For this review, take the finished solid that the model builds, in its own axes (mm). Give positions to 0.01 mm unless a question says otherwise; leave off trailing zeros. Loops run counter-clockwise (first coordinate to the right, second up) from the corner with the lowest first, then second, coordinate; pieces in that order, holes last. Notation, with made-up numbers: (-13.5, -7.75) -> (18.5, -7.75) arc R10 ccw to (18.5, 4.25) -> close; hole circle Ø8 at (37, 22.25). An arc over 180 degrees is marked (long way). Answer as CSV lines item,"result". Start each with the question number.
Item 1: For L1, parallel to Z at x = 136.5, y = 20.25; L2, parallel to Z at x = 135, y = 7.5; L3, parallel to Z at x = 72, y = 15, list the stretches that pass through material, from the lowest coordinate up. Write a range as from..to.
Item 2: Clearance check with flat-ended pins moving along their axes: P1, Ø0.8, axis at x = 211, y = 1, coming from the -Z side; P2, Ø4, axis at x = 289, z = 70, coming from the +Y side; P3, Ø0.5, axis at x = 345.5, y = 28.5, coming from the +Z side. State where each tip first meets the part, or that it passes through.
Item 3: The part is to be moulded in two halves that separate along Z. For faces 1 (the face through (303, 2.02, 60)), 2 (the face through (0, 15, 59)), 3 (the face through (303, 27.98, 60)), say which applies: +Z half, -Z half, draft (parallel to the pull), parting line (faces both ways), or undercut.
Item 4: Add section A-A on z = 28.5. State the section outline as (x, y) points, plus the area to 3 significant figures.
```python
from build123d import *

# Parameters (mm, degrees)
SKETCH1_W           = 598.4875
SKETCH1_H           = 30
BOSS_EXTRUDE1_DEPTH = 119.5
FILLET1_R           = 2
CUT_EXTRUDE1_REACH  = 613.038
FILLET2_R           = 0.5
CUT_EXTRUDE2_REACH  = 613.038
SKETCH3_W           = 98.3
SKETCH3_H           = 2.02
FILLET3_R           = 0.5


with BuildPart() as part:
    # Sketch1 → Boss-Extrude1 (new body)
    with BuildSketch(Plane.XY):
        with Locations((299.24375, 15)):
            Rectangle(SKETCH1_W, SKETCH1_H)
    extrude(amount=BOSS_EXTRUDE1_DEPTH)

    # Fillet1
    fillet1_edges = [part.edges().sort_by_distance(p)[0] for p in [
        (299.24375, 0, 119.5),
        (299.24375, 0, 0),
        (299.24375, 30, 0),
        (299.24375, 30, 119.5),
    ]]
    fillet(fillet1_edges, radius=FILLET1_R)

    # Sketch2 → Cut-Extrude1 (cut, up to next)
    with BuildSketch(Plane(origin=(598.4875, 0, 0), x_dir=(0, 0, -1), z_dir=(1, 0, 0)), mode=Mode.PRIVATE) as cut_extrude1_sk1:
        with BuildLine():
            Line((-119.5, 19.4), (-119.5, 10.6))
            Line((-119.5, 10.6), (-117.978098197, 10.6))
            ThreePointArc((-117.978098197, 10.6), (-117.624544806, 10.453553391), (-117.478098197, 10.1))
            Line((-117.478098197, 10.1), (-117.478098197, 6.87))
            ThreePointArc((-117.478098197, 6.87), (-117.331651588, 6.516446609), (-116.978098197, 6.37))
            Line((-116.978098197, 6.37), (-114.998098197, 6.37))
            ThreePointArc((-114.998098197, 6.37), (-114.783369216, 6.418456575), (-114.610260359, 6.554434141))
            Line((-114.610260359, 6.554434141), (-111.107479321, 10.859434141))
            ThreePointArc((-111.107479321, 10.859434141), (-111.024191423, 11.0075469), (-110.995317159, 11.175))
            Line((-110.995317159, 11.175), (-110.995317159, 18.825))
            ThreePointArc((-110.995317159, 18.825), (-111.024191423, 18.9924531), (-111.107479321, 19.140565859))
            Line((-111.107479321, 19.140565859), (-114.610260359, 23.445565859))
            ThreePointArc((-114.610260359, 23.445565859), (-114.783369216, 23.581543425), (-114.998098197, 23.63))
            Line((-114.998098197, 23.63), (-116.978098197, 23.63))
            ThreePointArc((-116.978098197, 23.63), (-117.331651588, 23.483553391), (-117.478098197, 23.13))
            Line((-117.478098197, 23.13), (-117.478098197, 19.9))
            ThreePointArc((-117.478098197, 19.9), (-117.624544806, 19.546446609), (-117.978098197, 19.4))
            Line((-117.978098197, 19.4), (-119.5, 19.4))
        make_face()
    cut_extrude1_tool1 = extrude(cut_extrude1_sk1.sketch, amount=-CUT_EXTRUDE1_REACH, mode=Mode.PRIVATE) & part.part
    cut_extrude1 = cut_extrude1_tool1.solids().sort_by_distance((598.4875, 15, 115.219459))[0]
    add(cut_extrude1, mode=Mode.SUBTRACT)

    # Mirror1: Cut-Extrude1 across plane
    add(cut_extrude1.mirror(Plane(origin=(0, 0, 59.75), x_dir=(1, 0, 0), z_dir=(0, 0, -1))), mode=Mode.SUBTRACT)

    # Fillet2
    fillet2_edges = [part.edges().sort_by_distance(p)[0] for p in [
        (299.24375, 10.6, 119.5),
        (299.24375, 19.4, 119.5),
    ]]
    fillet(fillet2_edges, radius=FILLET2_R)

    # Sketch3 → Cut-Extrude2 (cut, up to next)
    with BuildSketch(Plane(origin=(598.4875, 0, 0), x_dir=(0, 0, -1), z_dir=(1, 0, 0)), mode=Mode.PRIVATE) as cut_extrude2_sk1:
        with Locations((-59.75, 28.99)):
            Rectangle(SKETCH3_W, SKETCH3_H)
    cut_extrude2_tool1 = extrude(cut_extrude2_sk1.sketch, amount=-CUT_EXTRUDE2_REACH, mode=Mode.PRIVATE) & part.part
    cut_extrude2 = cut_extrude2_tool1.solids().sort_by_distance((598.4875, 28.99, 59.75))[0]
    add(cut_extrude2, mode=Mode.SUBTRACT)

    # Mirror2: Cut-Extrude2 across plane
    add(cut_extrude2.mirror(Plane.ZX.offset(15)), mode=Mode.SUBTRACT)

    # Fillet3
    fillet3_edges = [part.edges().sort_by_distance(p)[0] for p in [
        (299.24375, 30, 108.9),
        (299.24375, 30, 10.6),
        (299.24375, 0, 108.9),
        (299.24375, 0, 10.6),
    ]]
    fillet(fillet3_edges, radius=FILLET3_R)


solid = part.part
```
Computed values:
1,L1,"0..2.02, 7.49..112.01, 117.48..119.5"
1,L2,"0..2.02, 5.66..113.84, 117.48..119.5"
1,L3,"8.5..111"
2,P1,"z = 0.09"
2,P2,"y = 27.98"
2,P3,"z = 119.48"
3,face 1,"undercut"
3,face 2,"draft"
3,face 3,"undercut"
4,outline,"(0, 2.02) -> (598.49, 2.02) -> (598.49, 27.98) -> (0, 27.98) -> close"
4,area,"15,500 mm²"
